Work out the finished part from the listing and answer in its coordinate system (mm). A direction names the side the tool comes from. Give positions to 0.01 mm unless a question says otherwise; leave off trailing zeros. Loops run counter-clockwise (first coordinate to the right, second up) from the corner with the lowest first, then second, coordinate; pieces in that order, holes last. Notation, with made-up numbers: (87.25, 53.25) - (99.25, 53.25) arc R28 ccw to (99.25, 84.25) - close; hole circle Ø6 at (12, 71.25). An arc over 180 degrees is marked (long way). One line per item, written item: value.
Autodesk Inventor part; units mm, degrees
ref_plane "YZ Plane" through (0, 0, 0) normal (1, 0, 0) x (0, 1, 0)
ref_plane "XZ Plane" through (0, 0, 0) normal (0, 1, 0) x (-1, 0, 0)
ref_plane "XY Plane" through (0, 0, 0) normal (0, 0, 1) x (1, 0, 0)
ref_plane "Work Plane1" through (0, 0, 0) normal (0, 0, 1) x (1, 0, 0)
sketch "Sketch1" plane through (0, 0, 0) normal (0, 0, 1) x (1, 0, 0)
  line L0 (40, 0) -> (34, 0)
  line L1 (40, 0) -> (40, 260)
  line L2 (40, 260) -> (34, 260)
  line L3 (34, 0) -> (34, 260)
  line L4 (0, 0) -> (6, 0)
  line L5 (6, 0) -> (6, 260)
  line L6 (0, 260) -> (6, 260)
  line L7 (0, 0) -> (0, 260)
  line L8 (90, 15.4736) -> (-7, 15.4736)
  line L9 (-7, 15.4736) -> (-7, 85.4736)
  line L10 (-7, 85.4736) -> (90, 85.4736)
  line L11 (90, 85.4736) -> (90, 15.4736)
  line L12 (90, 85.4736) -> (-7, 15.4736) construction
  line L13 (90, 15.4736) -> (-7, 85.4736) construction
  line L14 (14, 0) -> (26, 0) construction
  line L15 (26, 0) -> (26, 260) construction
  line L16 (14, 260) -> (26, 260) construction
  line L17 (14, 0) -> (14, 260) construction
  circle A0 centre (-2, 25.4736) radius 2.45
  circle A1 centre (-2, 75.4736) radius 2.45
  circle A2 centre (51.5, 75.4736) radius 2.45
  circle A3 centre (51.5, 25.4736) radius 2.45
  line L18 (40, 40.4736) -> (-160, 40.4736)
  line L19 (40, 60.4736) -> (-160, 60.4736)
  circle A4 centre (-2, 25.4736) radius 2.45 construction
  circle A5 centre (-2, 75.4736) radius 2.45 construction
  line L20 (-7, 67.4547) -> (-7, 33.4924)
  dimension "d0" = 50
  dimension "d2" = 70
  dimension "d3" = 4.9
  dimension "d4" = 4.9
  dimension "d5" = 4.9
  dimension "d6" = 4.9
  dimension "d7" = 10
  dimension "d10" = 10
  dimension "d11" = 11.5
  dimension "d17" = 25
  dimension "d20" = 0
extrude "Extrusion1" add sketch "Sketch1" along normal blind 5 contours L8 L3 L18 L1 | L1 L10 L11 L8 | L8 L5 L18 L3 | L18 L3 L19 L1 | L18 L5 L19 L3 | L8 L7 A0 L18 L5 | L19 L3 L10 L1 | L19 L5 L10 L3 | L18 L7 L19 L5 | L8 L9 L18 L7 A0 | L19 L7 A1 L10 L5 | L18 L9 L19 L7 | L19 L9 L10 L7 A1
sketch "Sketch2" plane through (0, 0, 5) normal (0, 0, 1) x (1, 0, 0)
  circle A0 centre (69, 50.4736) radius 9.2
  circle A1 centre (84.5, 34.9736) radius 3
  circle A2 centre (53.5, 34.9736) radius 3
  circle A3 centre (53.5, 65.9736) radius 3
  line L0 (89.5, 67.2664) -> (89.5, 33.6807)
  arc A4 (89.5, 67.2664) -> (85.7929, 70.9736) centre (69, 50.4736) ccw
  line L1 (52.2071, 70.9736) -> (85.7929, 70.9736)
  arc A5 (52.2071, 70.9736) -> (48.5, 67.2664) centre (69, 50.4736) ccw
  line L2 (48.5, 33.6807) -> (48.5, 67.2664)
  arc A6 (48.5, 33.6807) -> (52.2071, 29.9736) centre (69, 50.4736) ccw
  line L3 (85.7929, 29.9736) -> (52.2071, 29.9736)
  arc A7 (85.7929, 29.9736) -> (89.5, 33.6807) centre (69, 50.4736) ccw
  circle A8 centre (84.5, 34.9736) radius 3
  circle A9 centre (53.5, 34.9736) radius 3
  circle A10 centre (84.5, 65.9736) radius 3
  circle A11 centre (69, 50.4736) radius 4
  circle A12 centre (53.5, 65.9736) radius 3
  point P0 (0, 0)
extrude "Extrusion2" cut sketch "Sketch2" against normal through all contours A0 | A11
sketch "Sketch3" plane through (0, 0, 5) normal (0, 0, 1) x (1, 0, 0)
  point P0 (0, 0)
sketch "Sketch4" plane through (0, 0, 5) normal (0, 0, 1) x (1, 0, 0)
  line L0 (89.5, 67.2664) -> (89.5, 33.6807)
  arc A0 (89.5, 67.2664) -> (85.7929, 70.9736) centre (69, 50.4736) ccw
  line L1 (52.2071, 70.9736) -> (85.7929, 70.9736)
  arc A1 (52.2071, 70.9736) -> (48.5, 67.2664) centre (69, 50.4736) ccw
  line L2 (48.5, 33.6807) -> (48.5, 67.2664)
  arc A2 (48.5, 33.6807) -> (52.2071, 29.9736) centre (69, 50.4736) ccw
  line L3 (85.7929, 29.9736) -> (52.2071, 29.9736)
  arc A3 (85.7929, 29.9736) -> (89.5, 33.6807) centre (69, 50.4736) ccw
  circle A4 centre (84.5, 34.9736) radius 3
  circle A5 centre (53.5, 34.9736) radius 3
  circle A6 centre (84.5, 65.9736) radius 3
  circle A7 centre (69, 50.4736) radius 4
  circle A8 centre (53.5, 65.9736) radius 3
  circle A9 centre (69, 50.4736) radius 9.2
  line L4 (90, 85.4736) -> (90, 15.4736)
  line L5 (48, 29.9736) -> (90, 29.9736)
  line L6 (90, 29.9736) -> (90, 70.9736)
  line L7 (90, 70.9736) -> (48, 70.9736)
  line L8 (48, 29.9736) -> (90, 70.9736) construction
  line L9 (90, 29.9736) -> (48, 70.9736) construction
  arc A10 (69, 38.8858) -> (69, 62.0613) centre (69, 50.4736) ccw
  line L10 (69, 38.8858) -> (48, 38.8858)
  line L11 (48, 62.0613) -> (69, 62.0613)
  line L12 (48, 70.9736) -> (48, 62.0613)
  line L13 (48, 38.8858) -> (48, 29.9736)
  line L14 (69, 62.0613) -> (69, 46.4736)
  line L15 (69, 41.2736) -> (69, 38.8858)
  point P0 (0, 0)
extrude "Extrusion3" add sketch "Sketch4" along normal blind 20 contours A0 L7 L4 L5 A3 L0 | L0 A3 L3 A2 L2 L10 A10 L11 A1 L1 A0 | A1 L2 L11 L12 L7 | L5 L13 L10 L2 A2 | A4 | A5 | A6 | A8
fillet "Fillet1" radius 5 8 edges at (90, 85.4736, 2.5) (-7, 85.4736, 2.5) (-7, 15.4736, 2.5) (90, 15.4736, 2.5) (48, 29.9736, 15) (90, 29.9736, 15) (48, 70.9736, 15) (90, 70.9736, 15)
sketch "Sketch5" plane through (0, 0, 0) normal (0, 0, -1) x (-1, 0, 0)
  line L0 (-40, 40.4736) -> (-40, 46.4736)
  line L1 (-40, 46.4736) -> (160, 46.4736)
  line L2 (160, 40.4736) -> (160, 46.4736)
  line L3 (-40, 40.4736) -> (160, 40.4736)
  line L4 (-40, 54.4736) -> (-40, 60.4736)
  line L5 (-40, 60.4736) -> (160, 60.4736)
  line L6 (160, 54.4736) -> (160, 60.4736)
  line L7 (-40, 54.4736) -> (160, 54.4736)
  circle A0 centre (12.6673, 50.4736) radius 1.45
  circle A1 centre (-27.3327, 50.4736) radius 1.45
  circle A2 centre (-7.3327, 50.4736) radius 1.45
  circle A3 centre (-47.3327, 50.4736) radius 1
  point P0 (0, 0)
  dimension "d24" = 2.9
  dimension "d25" = 2.9
  dimension "d26" = 2.9
  dimension "d27" = 4
  dimension "d28" = 4
  dimension "d29" = 4
  dimension "d30" = 20
  dimension "d31" = 20
  dimension "d39" = 2
  dimension "d40" = 4
  dimension "d41" = 20
hole "Hole1" at (-12.6673, 50.4736, 0) at (47.3327, 50.4736, 0) direction (0, 0, 1) diameter 2.9 end through all counterbore diameter 7 counterbore depth 3
sketch "Sketch6" plane through (0, 0, 0) normal (0, 0, -1) x (-1, 0, 0)
  line L0 (-52.2071, 29.9736) -> (-85.7929, 29.9736)
  arc A0 (-52.2071, 29.9736) -> (-48.5, 33.6807) centre (-69, 50.4736) ccw
  line L1 (-48.5, 67.2664) -> (-48.5, 33.6807)
  arc A1 (-48.5, 67.2664) -> (-52.2071, 70.9736) centre (-69, 50.4736) ccw
  line L2 (-85.7929, 70.9736) -> (-52.2071, 70.9736)
  arc A2 (-85.7929, 70.9736) -> (-89.5, 67.2664) centre (-69, 50.4736) ccw
  line L3 (-89.5, 33.6807) -> (-89.5, 67.2664)
  arc A3 (-89.5, 33.6807) -> (-85.7929, 29.9736) centre (-69, 50.4736) ccw
  circle A4 centre (-84.5, 34.9736) radius 3
  circle A5 centre (-84.5, 65.9736) radius 3
  circle A6 centre (-53.5, 34.9736) radius 3
  circle A7 centre (-69, 50.4736) radius 4
  circle A8 centre (-53.5, 65.9736) radius 3
  point P0 (0, 0)
  point P1 (-84.6331, 35.182)
hole "Hole2" at (84.5, 65.9736, 0) at (53.5, 65.9736, 0) at (53.5, 34.9736, 0) at (84.5, 34.9736, 0) direction (0, 0, 1) diameter 2.8 end through all counterbore diameter 8 counterbore depth 20
pattern_linear "Rectangular Pattern1" count 7 spacing 10 along (-1, 0, 0) of "Hole1"
equation "\"d3\" = d6"
equation "\"d4\" = d6"
equation "\"d5\" = d6"
properties part number "Neje_slide_y_20mmrod_upperplate"
1. Find the intervals of material crossed by line 1 along X through (y, z) = (32, 18.25); line 2 along Y through (x, z) = (51.5, 2.3); line 3 along Y through (x, z) = (60, 19.5), in increasing order.
Output:
line 1: x = 48.98 to 50.82, 56.18 to 81.82, 87.18 to 89.02
line 2: y = 15.47 to 23.02, 27.92 to 31.51, 38.44 to 62.51, 69.44 to 73.02, 77.92 to 85.47
line 3: y = 29.97 to 38.89, 62.06 to 70.97
2. Section D-D (z = 2) is taken. Count the separate pieces of the cut face and the enclosed holes in it, and give its area (3 significant figures).
Output:
separate pieces: 1
enclosed holes: 15
area: 6,000 mm²
3. The mould has two halves that part along X. Classify faces 4 (the cylindrical face through (85.74, 66.62, 22.54)), 5 (the flat face through (69, 70.974, 15)), 6 (the cylindrical face through (49.504, 69.548, 15.14)), 7 (the flat face through (90, 51, 10)): released by +X, released by -X, zero draft, split by the parting line, or undercut.
Output:
face 4: undercut
face 5: zero draft
face 6: released by -X
face 7: released by +X
4. For faces 1 (the cylindrical face through (18.67, 53.71, 1.52)), 2 (the cylindrical face through (-5.496, 84.048, 2.535)), 3 (the cylindrical face through (80.585, 50.728, 14.86)), determine the directions among +Z, -Z, +X, -X, +Y, -Y from which every point of the face is accessible in a straight line to the end or side of a thin tool.
Output:
face 1: -Z
face 2: +Z, -Z, -X, +Y
face 3: +Z, -X
5. Flat-ended cylindrical pins translate along their axes: pin 1 Ø3 at (x, y) = (84.5, 65.97) entering from -Z; pin 2 Ø3 at (y, z) = (33.5, 17.5) entering from -X; pin 3 Ø4 at (x, y) = (47.33, 50.47) entering from -Z. Find the tip coordinate at first contact, or state that the pin passes through.
Output:
pin 1: stops at z = 20
pin 2: stops at x = 48
pin 3: stops at z = 3
6. Section A-A (x = 73) is taken. Write down the section's boundary in (y, z).
Output:
outline: (15.47, 0) - (42.19, 0) - (42.19, 5) - (39.6, 5) - (39.6, 25) - (29.97, 25) - (29.97, 5) - (15.47, 5) - close; (58.76, 0) - (85.47, 0) - (85.47, 5) - (70.97, 5) - (70.97, 25) - (61.35, 25) - (61.35, 5) - (58.76, 5) - close
7. Section C-C (y = 57.5) is taken. Write down the section's boundary in (x, z).
Output:
outline: (-7, 0) - (63.06, 0) - (63.06, 5) - (-7, 5) - close; (74.94, 0) - (90, 0) - (90, 25) - (78.21, 25) - (78.21, 5) - (74.94, 5) - close
